Input: dimensioned drawing with shaded views. Units: mm. Origin: part minimum x, y, z. A direction names the side the tool comes from. Round coordinates to 2 decimals unless told otherwise and drop trailing zeros. Loops run counter-clockwise (first coordinate to the right, second up) from the corner with the lowest first, then second, coordinate; pieces in that order, holes last.
1) First-contact query: pin 1 (3 mm diameter, centred on y = 8, z = 2, fed in from +X); pin 2 (3 mm diameter, centred on y = 6.5, z = 7.5, fed in from -X); pin 3 (6 mm diameter, centred on x = 26, z = 8.5, fed in from +Y). Flat tips, straight axial feed; report the tip coordinate or a pass-through.
2) Section B-B, the plane z = 6. Return loops of the section in (x, y), and give its area (3 significant figures).
3) Section A-A, the plane y = 9.3. Return loops of the section in (x, z).
4) Section C-C, the plane x = 30. Return loops of the section in (y, z).
5) Access query for the marked faces 5, 6 and 7. Directions: +Z, -Z, +X, -X, +Y, -Y. A direction counts if a zero-diameter tool reaches every point of the face in a straight line with its end or side. Return the directions, or none.
6) Ray query, line 1 along X through (y, z) = (9.5, 11.5); line 2 along Y through (x, z) = (3.5, 9.5); line 3 along Y through (x, z) = (18.95, 6). Return the intervals inside material, ascending.
7) Draft query along X for the marked faces 1, 2, 3 and 4. Return one class per face: pulls with the +X half, pulls with the -X half, needs draft (parallel to the pull), parting line crosses it, or undercut.
8) Section D-D, the plane z = 2. Return loops of the section in (x, y).
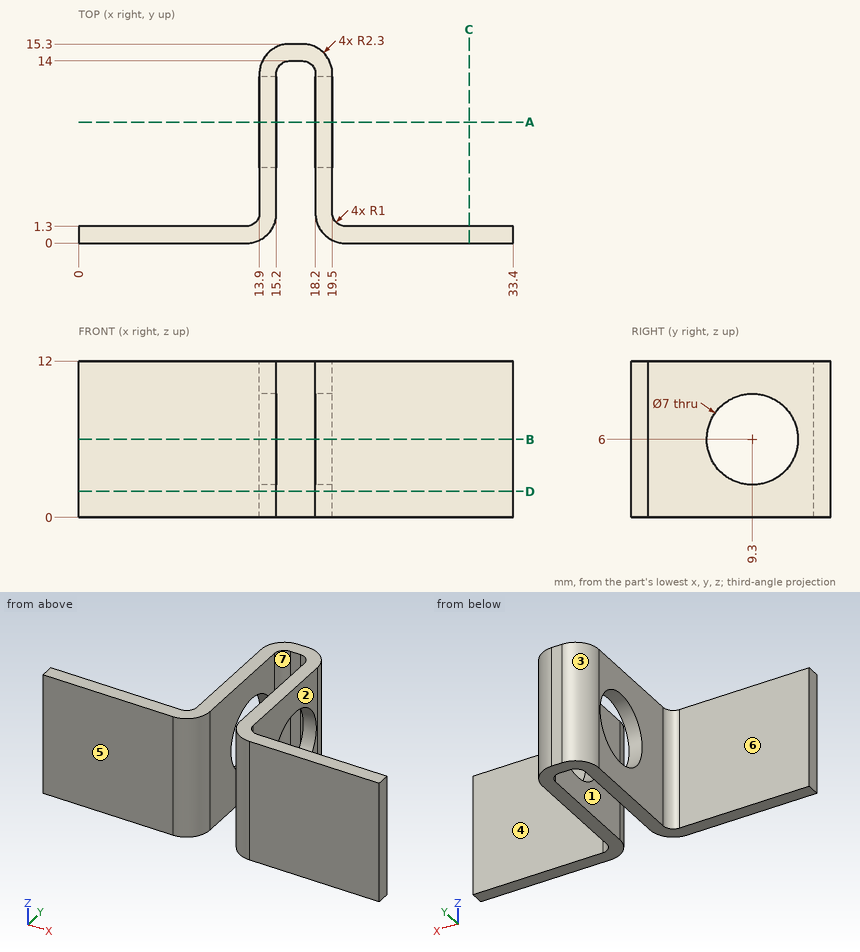
Final values:
1. pin 1: stops at x = 19.5
1. pin 2: stops at x = 13.9
1. pin 3: stops at y = 1.3
2. outline: (0, 0) - (12.9, 0) arc R2.3 ccw to (15.2, 2.3) - (15.2, 5.8) - (13.9, 5.8) - (13.9, 2.3) arc R1 cw to (12.9, 1.3) - (0, 1.3) - close; (13.9, 12.8) - (15.2, 12.8) - (15.2, 13) arc R1 cw to (16.2, 14) - (17.2, 14) arc R1 cw to (18.2, 13) - (18.2, 12.8) - (19.5, 12.8) - (19.5, 13) arc R2.3 ccw to (17.2, 15.3) - (16.2, 15.3) arc R2.3 ccw to (13.9, 13) - close; (18.2, 2.3) arc R2.3 ccw to (20.5, 0) - (33.4, 0) - (33.4, 1.3) - (20.5, 1.3) arc R1 cw to (19.5, 2.3) - (19.5, 5.8) - (18.2, 5.8) - close
2. area: 57.9 mm2
3. outline: (13.9, 0) - (15.2, 0) - (15.2, 2.5) - (13.9, 2.5) - close; (13.9, 9.5) - (15.2, 9.5) - (15.2, 12) - (13.9, 12) - close; (18.2, 0) - (19.5, 0) - (19.5, 2.5) - (18.2, 2.5) - close; (18.2, 9.5) - (19.5, 9.5) - (19.5, 12) - (18.2, 12) - close
4. outline: (0, 0) - (1.3, 0) - (1.3, 12) - (0, 12) - close
5. face 5: +Z, -Z, +X, -X, -Y
5. face 6: +Z, -Z, -X, +Y
5. face 7: +Z, -Z, -Y
6. line 1: x = 13.9 to 15.2, 18.2 to 19.5
6. line 2: y = 0 to 1.3
6. line 3: y = 0.6 to 5.8, 12.8 to 14.49
7. face 1: undercut
7. face 2: pulls with the +X half
7. face 3: pulls with the -X half
7. face 4: needs draft
8. outline: (0, 0) - (12.9, 0) arc R2.3 ccw to (15.2, 2.3) - (15.2, 13) arc R1 cw to (16.2, 14) - (17.2, 14) arc R1 cw to (18.2, 13) - (18.2, 2.3) arc R2.3 ccw to (20.5, 0) - (33.4, 0) - (33.4, 1.3) - (20.5, 1.3) arc R1 cw to (19.5, 2.3) - (19.5, 13) arc R2.3 ccw to (17.2, 15.3) - (16.2, 15.3) arc R2.3 ccw to (13.9, 13) - (13.9, 2.3) arc R1 cw to (12.9, 1.3) - (0, 1.3) - close
